```python
from build123d import *

# Parameters (mm, degrees)
F0_W     = 24.116488
F0_H     = 49.084154
F1_DEPTH = 8.382
F2_SIZE  = 6.35
F3_SIZE  = 6.604
F4_R     = 5.788051
F5_DEPTH = 9.144
F7_DEPTH = 0.508
F8_SIZE  = 1.1938


with BuildPart() as f1:
    # F0 (on Top) → F1 (new body)
    with BuildSketch(Plane.XY):
        Rectangle(F0_W, F0_H)
    extrude(amount=F1_DEPTH)

    # F2
    f2_edges = [f1.edges().sort_by_distance(p)[0] for p in [
        (0, -24.542077, 0),
    ]]
    chamfer(f2_edges, length=F2_SIZE)

    # F3
    f3_edges = [f1.edges().sort_by_distance(p)[0] for p in [
        (0, 24.542077, 0),
    ]]
    chamfer(f3_edges, length=F3_SIZE)

    # F4 (on Top) → F5 (join)
    with BuildSketch(Plane.XY):
        Circle(F4_R)
    extrude(amount=F5_DEPTH)

    # F6 (on face) → F7 (join)
    with BuildSketch(Plane.XY.offset(8.382)):
        Polygon((-8.432594, -21.930741), (-7.237773, -21.930741), (-6.392907, -21.085875), (-6.392907, -19.891055), (-7.237773, -19.046189), (-8.432594, -19.046189), (-9.277459, -19.891055), (-9.277459, -21.085875), align=None)
    extrude(amount=F7_DEPTH)

    # F8
    f8_edges = [f1.edges().sort_by_distance(p)[0] for p in [
        (0, -24.542077, 8.382),
    ]]
    chamfer(f8_edges, length=F8_SIZE)


solid = f1.part
```
Input: part model. Units: mm. Frame: model coordinates. A direction names the side the tool comes from. Give positions to 0.01 mm unless a question says otherwise; leave off trailing zeros. Loops run counter-clockwise (first coordinate to the right, second up) from the corner with the lowest first, then second, coordinate; pieces in that order, holes last. Notation, with made-up numbers: M 63.5,34 L 111.5,34 A10 cw 111.5,47 Z; hole C 14.25,-24.5 d4. An arc over 180 degrees is marked long. Answer as CSV lines item,"result". Start each with the question number.
1. Line query: L1, parallel to Z at x = -1.5, y = 14.5; L2, parallel to Y at x = -9, z = 8.75; L3, parallel to Y at x = 6, z = 8.25. Output: solid intervals per line, ascending.
2. Section C-C on x = 6.25. Return loops of the section in (y, z), plus the area to 3 significant figures.
3. Section A-A on x = 0. Return loops of the section in (y, z).
4. Reachability of faces 1 (the face through (-8.861, -21.502, 8.632)), 2 (the face through (-6.809, -19.475, 8.632)), 3 (the face through (-1.25, -5.65, 8.76)), 4 (the face through (-6.821, -21.514, 8.632)), 5 (the face through (-8.849, -19.463, 8.632)) from +Z, -Z, +X, -X, +Y, -Y: full face, straight path, thin tool, end or side. Return the list, or none.
5. Section D-D on z = 1.5. Return loops of the section in (x, y).
6. Section B-B on y = 0. Return loops of the section in (x, z).
7. Pin query (flat end, axial travel): P1, Ø3, axis at x = -8, y = -21, coming from the +Z side; P2, Ø12, axis at x = -9, y = -10, coming from the +Z side; P3, Ø0.6, axis at x = -8, z = 8.5, coming from the +Y side; P4, Ø0.6, axis at y = -20.5, z = 9, coming from the +X side. Return the tip coordinate at first contact, or that it passes through.
Computed values:
1,L1,"z = 0 to 8.38"
1,L2,"y = -21.36 to -19.61"
1,L3,"y = -23.48 to 24.54"
2,outline,"M -24.54,6.35 L -18.19,0 L 17.94,0 L 24.54,6.6 L 24.54,8.38 L -23.35,8.38 L -24.54,7.19 Z"
2,area,"369 mm²"
3,outline,"M -24.54,6.35 L -18.19,0 L 17.94,0 L 24.54,6.6 L 24.54,8.38 L 5.79,8.38 L 5.79,9.14 L -5.79,9.14 L -5.79,8.38 L -23.35,8.38 L -24.54,7.19 Z"
4,face 1,"+Z, -X, -Y"
4,face 2,"+Z, +X, +Y"
4,face 3,"+Z"
4,face 4,"+Z, +X, -Y"
4,face 5,"+Z, -X, +Y"
5,outline,"M -12.06,-19.69 L 12.06,-19.69 L 12.06,19.44 L -12.06,19.44 Z"
6,outline,"M -12.06,0 L 12.06,0 L 12.06,8.38 L 5.79,8.38 L 5.79,9.14 L -5.79,9.14 L -5.79,8.38 L -12.06,8.38 Z"
7,P1,"stops at z = 8.89"
7,P2,"stops at z = 8.38"
7,P3,"stops at y = 24.54"
7,P4,"stops at x = -6.39"
